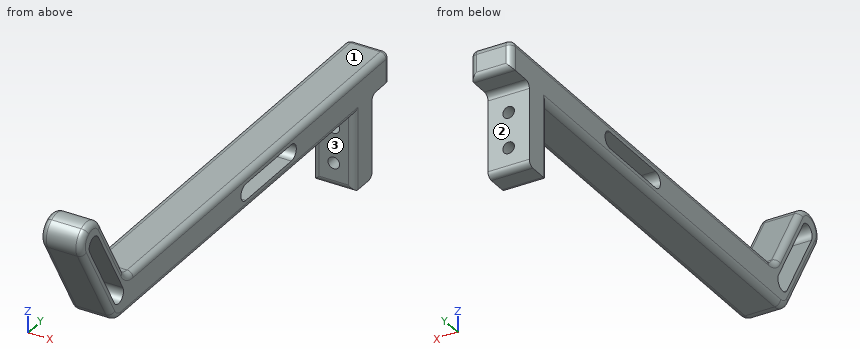
```python
from build123d import *

# Parameters (mm, degrees)
BOSS_EXTRUDE1_DEPTH     = 8.89
CUT_EXTRUDE1_DEPTH      = 10.16
CUT_EXTRUDE2_DEPTH      = 10.16
TAP_DRILL_FOR_M3_TAP1_D = 2.5
FILLET5_R               = 1.27
FILLET6_R               = 3.81
FILLET7_R               = 1.27


with BuildPart() as part:
    # Sketch1 → Boss-Extrude1 (new body)
    with BuildSketch(Plane(origin=(0, 0, 0), x_dir=(0, 0, -1), z_dir=(1, 0, 0))):
        Polygon((-2.31554316, -8.033202767), (20.781354359, 5.301797233), (20.781354359, 92.169797233), (37.291354359, 92.169797233), (37.291354359, 98.519797233), (19.511354359, 98.519797233), (19.511354359, 104.869797233), (13.161354359, 104.869797233), (13.161354359, 9.701206284), (-6.12554316, -1.43408919), align=None)
    extrude(amount=BOSS_EXTRUDE1_DEPTH)

    # Sketch2 → Cut-Extrude1 (cut)
    with BuildSketch(Plane(origin=(8.89, 0, 0), x_dir=(0, 0, -1), z_dir=(1, 0, 0))):
        with BuildLine():
            Line((1.067865891, -3.733439147), (16.465797571, 5.156560853))
            ThreePointArc((16.465797571, 5.156560853), (17.116590739, 7.585354021), (14.687797571, 8.236147189))
            Line((14.687797571, 8.236147189), (-0.710134109, -0.653852811))
            ThreePointArc((-0.710134109, -0.653852811), (-1.360927276, -3.082645979), (1.067865891, -3.733439147))
        make_face()
    extrude(amount=-CUT_EXTRUDE1_DEPTH, mode=Mode.SUBTRACT)

    # Sketch3 → Cut-Extrude2 (cut)
    with BuildSketch(Plane(origin=(8.89, 0, 0), x_dir=(0, 0, -1), z_dir=(1, 0, 0))):
        with BuildLine():
            Line((15.193354359, 69.309797233), (15.193354359, 52.799797233))
            ThreePointArc((15.193354359, 52.799797233), (16.971354359, 51.021797233), (18.749354359, 52.799797233))
            Line((18.749354359, 52.799797233), (18.749354359, 69.309797233))
            ThreePointArc((18.749354359, 69.309797233), (16.971354359, 71.087797233), (15.193354359, 69.309797233))
        make_face()
    extrude(amount=-CUT_EXTRUDE2_DEPTH, mode=Mode.SUBTRACT)

    # Tap Drill for M3 Tap1 (through all)
    with Locations(Plane(origin=(0, 98.519797233, 0), x_dir=(1, 0, 0), z_dir=(0, 1, 0))):
        with Locations((4.445, 32.211354359), (4.445, 24.591354359)):
            Hole(TAP_DRILL_FOR_M3_TAP1_D / 2)

    # Fillet5
    fillet5_edges = [part.edges().sort_by_distance(p)[0] for p in [
        (4.445, 98.519797233, -19.511354359),
        (4.445, 98.519797233, -37.291354359),
    ]]
    fillet(fillet5_edges, radius=FILLET5_R)

    # Fillet6
    fillet6_edges = [part.edges().sort_by_distance(p)[0] for p in [
        (4.445, 9.701206284, -13.161354359),
        (4.445, 5.301797233, -20.781354359),
        (4.445, -8.033202767, 2.31554316),
        (4.445, -1.43408919, 6.12554316),
    ]]
    fillet(fillet6_edges, radius=FILLET6_R - 0.0001)  # a hair under: the kernel refuses the full size

    # Fillet7
    fillet7_edges = [part.edges().sort_by_distance(p)[0] for p in [
        (8.89, 5.596494023, -20.270924545),
        (0, 9.995903075, -12.650924545),
        (8.89, 9.995903075, -12.650924545),
        (0, 104.869797233, -16.336354359),
        (0, 92.169797233, -29.036354359),
        (8.89, 92.169797233, -29.036354359),
        (4.445, 104.869797233, -13.161354359),
        (4.445, 104.869797233, -19.511354359),
        (4.445, 92.169797233, -37.291354359),
        (8.89, 104.869797233, -16.336354359),
        (8.89, 58.385325154, -13.161354359),
        (0, 4.536121849, -4.215165693),
        (8.89, 4.536121849, -4.215165693),
        (0, 49.835620628, -20.781354359),
        (8.89, 49.835620628, -20.781354359),
        (0, -0.963139465, -9.930165693),
        (0, -1.842534696, 4.601203779),
        (0, -6.508863387, 1.907097654),
        (0, 5.596494023, -20.270924545),
        (0, 58.385325154, -13.161354359),
        (8.89, -0.963139465, -9.930165693),
        (8.89, -1.842534696, 4.601203779),
        (8.89, -6.508863387, 1.907097654),
    ]]
    fillet(fillet7_edges, radius=FILLET7_R)


solid = part.part
```
Verification items for the finished model (mm, model axes). Face numbers are marked on the shaded views. A direction names the side the tool comes from. Coordinates: 2 decimals unless noted, no trailing zeros. Loops run counter-clockwise (first coordinate to the right, second up) from the corner with the lowest first, then second, coordinate; pieces in that order, holes last. Notation, with made-up numbers: (-27, -38) -> (-7, -38) arc R28 ccw to (-7, -18) -> close; hole circle Ø11 at (56, 12.25). An arc over 180 degrees is marked (long way). Answer in a Markdown table with one row per item. Add a question column.
1. Material ranges on probe 1 along Y at (x, z) = (2.25, -15.5); probe 2 along Z at (x, y) = (5, 94.5); probe 3 along Y at (x, z) = (7, -32), recorded low to high. Write a range as [from, to].
2. Access from +Z, -Z, +X, -X, +Y, -Y to the whole of each face (thin tool, end or side, straight path). Record for the marked faces 1, 2 and 3.
3. Section check B-B, the plane y = 83. Enter the section's corners in (x, z).
4. Section check A-A, the plane y = 67. Enter the section's corners in (x, z), then the cut area to 3 significant figures.
5. Section check C-C, the plane z = -27. Enter the section's corners in (x, y).
6. Section check D-D, the plane x = 4.25. Give the number of separate pieces and of enclosed holes in the cut face, then the cut area to 3 significant figures.
7. Depth check by flat-ended pin: P1, Ø1, axis at x = 7, y = 93, coming from the +Z side; P2, Ø10, axis at y = 88.5, z = -22, coming from the -X side; P3, Ø3, axis at x = 4.44, z = -24.59, coming from the +Y side; P4, Ø3, axis at x = 4, z = -29, coming from the -Y side. Enter the tip coordinate at first touch or a pass-through.
Derived:
| question | item | result |
|---|---|---|
| 1 | probe 1 | y = [2.25, 4.6], [8.47, 51.8], [70.31, 104.87] |
| 1 | probe 2 | z = [-37.29, -33.33], [-31.09, -25.71], [-23.47, -13.16] |
| 1 | probe 3 | y = [92.17, 98.52] |
| 2 | face 1 | +Z, +X, -X, +Y |
| 2 | face 2 | -Z, +X, -X, +Y |
| 2 | face 3 | -Z, +X, -X, -Y |
| 3 | outline | (0, -19.51) arc R1.27 ccw to (1.27, -20.78) -> (7.62, -20.78) arc R1.27 ccw to (8.89, -19.51) -> (8.89, -14.43) arc R1.27 ccw to (7.62, -13.16) -> (1.27, -13.16) arc R1.27 ccw to (0, -14.43) -> close |
| 4 | outline | (0, -19.51) arc R1.27 ccw to (1.27, -20.78) -> (7.62, -20.78) arc R1.27 ccw to (8.89, -19.51) -> (8.89, -18.75) -> (0, -18.75) -> close; (0, -15.19) -> (8.89, -15.19) -> (8.89, -14.43) arc R1.27 ccw to (7.62, -13.16) -> (1.27, -13.16) arc R1.27 ccw to (0, -14.43) -> close |
| 4 | area | 34.7 mm² |
| 5 | outline | (0, 93.44) arc R1.27 ccw to (1.27, 92.17) -> (7.62, 92.17) arc R1.27 ccw to (8.89, 93.44) -> (8.89, 98.52) -> (0, 98.52) -> close |
| 6 | separate pieces | 3 |
| 6 | enclosed holes | 2 |
| 6 | area | 845 mm² |
| 7 | P1 | stops at z = -13.16 |
| 7 | P2 | stops at x = 0 |
| 7 | P3 | stops at y = 98.52 |
| 7 | P4 | stops at y = 92.17 |
